Geometry check sheet. Reference: the model listing, model coordinates, mm. Face numbers are marked on the shaded views. A direction names the side the tool comes from. Round coordinates to 2 decimals unless told otherwise and drop trailing zeros. Loops run counter-clockwise (first coordinate to the right, second up) from the corner with the lowest first, then second, coordinate; pieces in that order, holes last. Notation, with made-up numbers: (-35, 70) -> (-30, 70) arc R20 cw to (-30, 77) -> close; hole circle Ø6 at (87.5, 31.25). An arc over 180 degrees is marked (long way). Use a Markdown table: item, result. Add a question column.
Q1. Sectioned sample at A-A, the plane x = -56. Enter the section's corners in (y, z) (3 decimals), then the cut area to 3 significant figures.
Q2. Sectioned sample at C-C, the plane z = 36. Enter the section's corners in (x, y).
Q3. Gauge pin test, flat ends, axial feed: P1, Ø10, axis at y = 38.5, z = 26.5, coming from the -X side; P2, Ø2, axis at x = -48, y = 26.5, coming from the +Z side (3 decimals). Record the tip position at first contact, or that the pin passes through.
Q4. Sectioned sample at B-B, the plane y = 47. Enter the section's corners in (x, z) (3 decimals), then the cut area to 3 significant figures.
Q5. Set-up check for the marked faces 1, 2 and 3: record each of +Z, -Z, +X, -X, +Y, -Y from which the full face is reachable in a straight line by a thin tool's end or side.
Q6. Sectioned sample at D-D, the plane y = 31.5. Enter the section's corners in (x, z) (3 decimals).
Q7. Material ranges on L1, parallel to Z at x = -72, y = 50 (3 decimals); L2, parallel to X at y = 42.5, z = 42.5, recorded low to high.
Q8. Release check for a two-part mould opening along X. For the marked faces 4, 5, 6 and 7 record: released by +X, released by -X, zero draft, split by the parting line, or undercut.
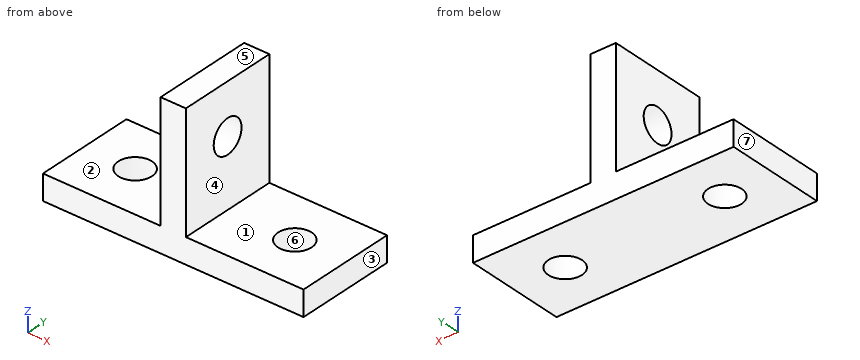
```python
from build123d import *

# Parameters (mm, degrees)
F0_W     = 98.425
F0_H     = 38.1
F1_DEPTH = 9.525
F3_D     = 12.7
F5_DEPTH = 44.45
F7_D     = 12.7


with BuildPart() as f1:
    # F0 (on Top) → F1 (new body)
    with BuildSketch(Plane.XY):
        with Locations((-27.238064, 36.847196)):
            Rectangle(F0_W, F0_H)
    extrude(amount=F1_DEPTH)

    # F3 (through all)
    with Locations(Plane.XY.offset(9.525)):
        with Locations((-57.400564, 36.847196), (2.924436, 36.847196)):
            Hole(F3_D / 2)

    # F4 (on face) → F5 (join)
    with BuildSketch(Plane.XY.offset(9.525)):
        Polygon((-32.000564, 17.797196), (-27.238064, 17.797196), (-22.475564, 17.797196), (-22.475564, 55.897196), (-27.238064, 55.897196), (-32.000564, 55.897196), align=None)
    extrude(amount=F5_DEPTH)

    # F7 (through all)
    with Locations(Plane.YZ.offset(-22.475564)):
        with Locations((36.847196, 34.925)):
            Hole(F7_D / 2)


solid = f1.part
```
Values:
| question | item | result |
|---|---|---|
| 1 | outline | (17.797, 0) -> (30.654, 0) -> (30.654, 9.525) -> (17.797, 9.525) -> close; (43.041, 0) -> (55.897, 0) -> (55.897, 9.525) -> (43.041, 9.525) -> close |
| 1 | area | 245 mm^2 |
| 2 | outline | (-32, 17.8) -> (-22.48, 17.8) -> (-22.48, 30.59) -> (-32, 30.59) -> close; (-32, 43.11) -> (-22.48, 43.11) -> (-22.48, 55.9) -> (-32, 55.9) -> close |
| 3 | P1 | x = -32 |
| 3 | P2 | z = 9.525 |
| 4 | outline | (-76.451, 0) -> (21.974, 0) -> (21.974, 9.525) -> (-22.476, 9.525) -> (-22.476, 53.975) -> (-32.001, 53.975) -> (-32.001, 9.525) -> (-76.451, 9.525) -> close |
| 4 | area | 1,360 mm^2 |
| 5 | face 1 | +Z, +X, +Y, -Y |
| 5 | face 2 | +Z, -X, +Y, -Y |
| 5 | face 3 | +Z, -Z, +X, +Y, -Y |
| 6 | outline | (-76.451, 0) -> (-60.825, 0) -> (-60.825, 9.525) -> (-76.451, 9.525) -> close; (-53.976, 0) -> (-0.5, 0) -> (-0.5, 9.525) -> (-22.476, 9.525) -> (-22.476, 31.5) -> (-32.001, 31.5) -> (-32.001, 9.525) -> (-53.976, 9.525) -> close; (-32.001, 38.35) -> (-22.476, 38.35) -> (-22.476, 53.975) -> (-32.001, 53.975) -> close; (6.349, 0) -> (21.974, 0) -> (21.974, 9.525) -> (6.349, 9.525) -> close |
| 7 | L1 | 0 to 9.525 |
| 7 | L2 | -32 to -22.48 |
| 8 | face 4 | released by +X |
| 8 | face 5 | zero draft |
| 8 | face 6 | undercut |
| 8 | face 7 | released by -X |
